Here's how the part is built. I have some questions about the finished solid (model axes, mm). Give positions to 0.01 mm unless a question says otherwise; leave off trailing zeros. Write each loop counter-clockwise with the first axis right and the second up, starting at its lowest first coordinate (ties: lowest second). Pieces come first, ordered by that corner, then holes. Notation, with made-up numbers: (32, 1) -> (36, 1) arc R17 ccw to (36, 28) -> close; hole circle Ø4 at (-23.5, -37.75). An arc over 180 degrees is marked (long way). Use one line per item in the form item = value.
```python
from build123d import *

# Parameters (mm, degrees)
SKETCH1_W           = 9.525
SKETCH1_H           = 7.9375
BOSS_EXTRUDE1_DEPTH = 19.05


with BuildPart() as part:
    # Sketch1 → Boss-Extrude1 (new body)
    with BuildSketch(Plane(origin=(0, 0, 0), x_dir=(1, 0, 0), z_dir=(0, 1, 0))):
        Rectangle(SKETCH1_W, SKETCH1_H)
    extrude(amount=BOSS_EXTRUDE1_DEPTH)

    # Sketch3 → Revolve1 (revolve)
    with BuildSketch(Plane(origin=(0, 0, 0), x_dir=(0, 0, -1), z_dir=(1, 0, 0))):
        with BuildLine():
            Line((-3.96875, 14.2875), (-3.96875, 15.758974771))
            ThreePointArc((-3.96875, 15.758974771), (-5.009239789, 15.327989789), (-5.440224771, 14.2875))
            Line((-5.440224771, 14.2875), (-3.96875, 14.2875))
        make_face()
    revolve(axis=Axis((0, 14.2875, 3.96875), (0, 0, 1)))


solid = part.part
```
Q1. I want a section at D-D, the plane x = -4. Write out the boundary of the cut face in (y, z).
Result set:
outline = (0, -3.97) -> (19.05, -3.97) -> (19.05, 3.97) -> (0, 3.97) -> close
Q2. I want a section at C-C, the plane z = 4.5. Write out the boundary of the cut face in (x, y), and give its area (3 significant figures).
Result set:
outline = circle Ø2.74 at (0, 14.29)
area = 5.92 mm2
Q3. I want a section at A-A, the plane x = -0.5. Write out the boundary of the cut face in (y, z), and give its area (3 significant figures).
Result set:
outline = (0, -3.97) -> (19.05, -3.97) -> (19.05, 3.97) -> (15.67, 3.97) arc R1.38 ccw to (12.9, 3.97) -> (0, 3.97) -> close
area = 154 mm2
Q4. I want a section at B-B, the plane y = 6. Write out the boundary of the cut face in (x, z).
Result set:
outline = (-4.76, -3.97) -> (4.76, -3.97) -> (4.76, 3.97) -> (-4.76, 3.97) -> close
Q5. If I drill on line 1 along Z through (x, y) = (4.25, 6.5), over which ranges is the centre line in solid material (lowest first)? Write a range as from..to.
Result set:
line_1 = -3.97..3.97
